Source: CAD feature listing. Evaluate the final solid. Frame: model axes, mm. Give positions to 0.01 mm unless a question says otherwise; leave off trailing zeros. Loops run counter-clockwise (first coordinate to the right, second up) from the corner with the lowest first, then second, coordinate; pieces in that order, holes last.
```python
from build123d import *

# Parameters (mm, degrees)
SKETCH_R   = 35
SKETCH_R_2 = 5
PAD_DEPTH  = 10


with BuildPart() as part:
    # Sketch → Pad (new body)
    with BuildSketch(Plane.XY):
        with BuildLine():
            ThreePointArc((8.738871, 63.421137), (0.026212, 67.229999), (-8.689414, 63.427932))
            Line((-8.689414, 63.427932), (-38.097709, 31.714926))
            ThreePointArc((-38.097709, 31.714926), (-43.116334, 24.915646), (-46.50141, 17.172386))
            Line((-59.293751, -24.142484), (-46.50141, 17.172386))
            ThreePointArc((-59.293751, -24.142484), (-58.070122, -33.870995), (-49.949432, -39.366044))
            Line((-49.949432, -39.366044), (-7.319303, -46.662246))
            ThreePointArc((-7.319303, -46.662246), (-0.018435, -47.283947), (7.282915, -46.667939))
            Line((49.918721, -39.404981), (7.282915, -46.667939))
            ThreePointArc((49.918721, -39.404981), (58.043693, -33.916265), (59.274907, -24.188712))
            Line((46.514786, 17.136121), (59.274907, -24.188712))
            ThreePointArc((46.514786, 17.136121), (43.135749, 24.882018), (38.122428, 31.685209))
            Line((8.738871, 63.421137), (38.122428, 31.685209))
        make_face()
        Circle(SKETCH_R, mode=Mode.SUBTRACT)
        with Locations((-47.945296, -27.656311)):
            Circle(SKETCH_R_2, mode=Mode.SUBTRACT)
        with Locations((47.923716, -27.693689)):
            Circle(SKETCH_R_2, mode=Mode.SUBTRACT)
        with Locations((0.02158, 55.35)):
            Circle(SKETCH_R_2, mode=Mode.SUBTRACT)
    extrude(amount=PAD_DEPTH)


solid = part.part
```
(1) Section D-D, the plane x = 0. Return the cut outline in (y, z), then the cut area to 3 significant figures.
A:
outline: (-47.28, 0) - (-35, 0) - (-35, 10) - (-47.28, 10) - close; (35, 0) - (50.35, 0) - (50.35, 10) - (35, 10) - close; (60.35, 0) - (67.23, 0) - (67.23, 10) - (60.35, 10) - close
area: 345 mm2
(2) Section C-C, the plane z = 5. Return the cut outline in (x, y), then the cut area to 3 significant figures.
A:
outline: (-59.29, -24.14) arc R11.88 ccw to (-49.95, -39.37) - (-7.32, -46.66) arc R43.38 ccw to (7.28, -46.67) - (49.92, -39.4) arc R11.88 ccw to (59.27, -24.19) - (46.51, 17.14) arc R37.85 ccw to (38.12, 31.69) - (8.74, 63.42) arc R11.88 ccw to (-8.69, 63.43) - (-38.1, 31.71) arc R37.85 ccw to (-46.5, 17.17) - close; hole circle Ø10 at (-47.95, -27.66); hole circle Ø70 at (0, 0); hole circle Ø10 at (0.02, 55.35); hole circle Ø10 at (47.92, -27.69)
area: 5,260 mm2
(3) Section B-B, the plane x = 20. Return the cut outline in (y, z).
A:
outline: (-44.5, 0) - (-28.72, 0) - (-28.72, 10) - (-44.5, 10) - close; (28.72, 0) - (51.26, 0) - (51.26, 10) - (28.72, 10) - close
(4) Mould query, pull axis X, two halves, no side actions, for faces 1 (the cylindrical face through (0.16, 67.23, 4.93)), 2 (the cylindrical face through (52.54, -29.61, 4.93)), 3 (the flat face through (-23.19, 47.79, 4.93)), 4 (the cylindrical face through (-28, -21, 5)). Classes: pulls with the +X half, pulls with the -X half, needs draft (parallel to the pull), parting line crosses it, or undercut.
A:
face 1: parting line crosses it
face 2: undercut
face 3: pulls with the -X half
face 4: undercut
(5) Section A-A, the plane y = -10.5. Return the cut outline in (x, z), then the cut area to 3 significant figures.
A:
outline: (-55.07, 0) - (-33.39, 0) - (-33.39, 10) - (-55.07, 10) - close; (33.39, 0) - (55.05, 0) - (55.05, 10) - (33.39, 10) - close
area: 433 mm2
(6) Ray query, line 1 along X through (y, z) = (-25, 8.25); line 2 along X through (y, z) = (7, 4); line 3 along X through (y, z) = (57, 5.25). Return the intervals inside material, ascending.
A:
line 1: x = -59.52 to -52.18, -43.71 to -24.49, 24.49 to 43.71, 52.14 to 59.49
line 2: x = -49.65 to -34.29, 34.29 to 49.64
line 3: x = -14.65 to -4.7, 4.74 to 14.68
(7) First-contact query: pin 1 (6 mm diameter, centred on y = 46.5, z = 5.5, fed in from +X); pin 2 (5 mm diameter, centred on x = 23, z = 6.5, fed in from -Y); pin 3 (4 mm diameter, centred on x = 33.5, z = 9, fed in from -Y); pin 4 (12 mm diameter, centred on x = -24.5, y = -23, fed in from -Z). Flat tips, straight axial feed; report the tip coordinate or a pass-through.
A:
pin 1: stops at x = 27.18
pin 2: stops at y = -44.42
pin 3: stops at y = -42.54
pin 4: stops at z = 0
